Design review of the part built by this model. Coordinates are the model's own, in mm. A direction names the side the tool comes from. Coordinates: 2 decimals unless noted, no trailing zeros. Write each loop counter-clockwise with the first axis right and the second up, starting at its lowest first coordinate (ties: lowest second). Pieces come first, ordered by that corner, then holes. Notation, with made-up numbers: M 68.25,0 L 80.25,0 A29 cw 80.25,22 Z; hole C -36.75,30 d6. An arc over 180 degrees is marked long. One line per question, with ' | ' between items.
from build123d import *

# Parameters (mm, degrees)
SKETCH1_W               = 175
SKETCH1_H               = 80
BOSS_EXTRUDE1_DEPTH     = 7
SKETCH2_R               = 2
CUT_EXTRUDE1_DEPTH      = 10
SKETCH3_W               = 160
SKETCH3_H               = 52
CUT_EXTRUDE2_DEPTH      = 1
CUT_EXTRUDE3_DEPTH      = 10
SKETCH7_W               = 6
SKETCH7_H               = 15.226692755
SKETCH7_H_2             = 18
BOSS_EXTRUDE3_DEPTH     = 15
SKETCH8_R               = 2
CUT_EXTRUDE4_DEPTH      = 15
SKETCH9_W               = 20
SKETCH9_H               = 20
CUT_EXTRUDE5_DEPTH      = 15
SKETCH10_R              = 2
CUT_EXTRUDE7_DEPTH      = 51
CUT_EXTRUDE7_DEPTH_BACK = 31
SKETCH11_R              = 2
CUT_EXTRUDE8_DEPTH      = 10


with BuildPart() as part:
    # Sketch1 → Boss-Extrude1 (new body)
    with BuildSketch(Plane(origin=(0, 0, 0), x_dir=(1, 0, 0), z_dir=(0, 1, 0))):
        with Locations((-2.383449883, -6.993006993)):
            Rectangle(SKETCH1_W, SKETCH1_H)
    extrude(amount=BOSS_EXTRUDE1_DEPTH)

    # Sketch2 → Cut-Extrude1 (cut)
    with BuildSketch(Plane(origin=(0, 7, 0), x_dir=(1, 0, 0), z_dir=(0, 1, 0))):
        with Locations((-54.883449883, -32.893006993)):
            Circle(SKETCH2_R)
        with Locations((-2.383449883, -32.893006993)):
            Circle(SKETCH2_R)
        with Locations((50.116550117, -32.893006993)):
            Circle(SKETCH2_R)
    extrude(amount=-CUT_EXTRUDE1_DEPTH, mode=Mode.SUBTRACT)

    # Sketch3 → Cut-Extrude2 (cut)
    with BuildSketch(Plane(origin=(0, 7, 0), x_dir=(1, 0, 0), z_dir=(0, 1, 0))):
        with Locations((5.116550117, 7.006993007)):
            Rectangle(SKETCH3_W, SKETCH3_H)
    extrude(amount=-CUT_EXTRUDE2_DEPTH, mode=Mode.SUBTRACT)

    # Sketch6 → Cut-Extrude3 (cut)
    with BuildSketch(Plane(origin=(0, 6, 0), x_dir=(1, 0, 0), z_dir=(0, 1, 0))):
        Polygon((-70.883449883, 23.006993007), (-70.883449883, -18.993006993), (45.116550117, -18.993006993), (45.116550117, 23.006993007), (-9.883449883, 23.006993007), (-9.883449883, 28.006993007), (-70.883449883, 28.006993007), align=None)
    extrude(amount=-CUT_EXTRUDE3_DEPTH, mode=Mode.SUBTRACT)

    # Sketch7 → Boss-Extrude3 (add)
    with BuildSketch(Plane(origin=(0, 7, 0), x_dir=(1, 0, 0), z_dir=(0, 1, 0))):
        with Locations((-86.883449883, 25.39364663)):
            Rectangle(SKETCH7_W, SKETCH7_H)
        with Locations((-86.883449883, -32.993006993)):
            Rectangle(SKETCH7_W, SKETCH7_H_2)
    extrude(amount=BOSS_EXTRUDE3_DEPTH)

    # Sketch8 → Cut-Extrude4 (cut)
    with BuildSketch(Plane(origin=(-83.883449883, 0, 0), x_dir=(0, 0, -1), z_dir=(1, 0, 0))):
        with Locations((25.506993007, 14.5)):
            Circle(SKETCH8_R)
        with Locations((-32.993006993, 14.5)):
            Circle(SKETCH8_R)
    extrude(amount=-CUT_EXTRUDE4_DEPTH, mode=Mode.SUBTRACT)

    # Sketch9 → Cut-Extrude5 (cut)
    with BuildSketch(Plane.XZ):
        with Locations((75.116550117, 6.993006993)):
            Rectangle(SKETCH9_W, SKETCH9_H)
    extrude(amount=-CUT_EXTRUDE5_DEPTH, mode=Mode.SUBTRACT)

    # Sketch10 → Cut-Extrude7 (cut, two sides)
    with BuildSketch(Plane.XY.offset(-3.006993007)) as cut_extrude7_sk:
        with Locations((75.116550117, 3.5)):
            Circle(SKETCH10_R)
    extrude(amount=CUT_EXTRUDE7_DEPTH, mode=Mode.SUBTRACT)
    extrude(cut_extrude7_sk.sketch, amount=-CUT_EXTRUDE7_DEPTH_BACK, mode=Mode.SUBTRACT)

    # Sketch11 → Cut-Extrude8 (cut)
    with BuildSketch(Plane.XZ):
        with Locations((60.116550117, -23.006993007)):
            Circle(SKETCH11_R)
    extrude(amount=-CUT_EXTRUDE8_DEPTH, mode=Mode.SUBTRACT)


solid = part.part
1. Tool access review of faces 3 (the face through (-87, 14, 23.993)), 4 (the face through (-83.883, 12.7, -27)), 5 (the face through (-70.883, 3, -5)), 6 (the face through (28, 6, -24)): name each direction out of +Z, -Z, +X, -X, +Y, -Y from which nothing blocks a thin tool from reaching the whole face with its end or side.
Answer sheet:
face 3: +X, -X, +Y | face 4: +Z, -Z, +X, +Y | face 5: +Y, -Y | face 6: -Z, +X, +Y
2. Take a section at A-A (y = 9). Write out the cut boundary in (x, z).
Answer sheet:
outline: M -89.88,-33.01 L -83.88,-33.01 L -83.88,-17.78 L -89.88,-17.78 Z; M -89.88,23.99 L -83.88,23.99 L -83.88,41.99 L -89.88,41.99 Z
3. Take a section at B-B (x = -19). Write out the cut boundary in (y, z), then the cut area to 3 significant figures.
Answer sheet:
outline: M 0,-33.01 L 6,-33.01 L 6,-28.01 L 0,-28.01 Z; M 0,18.99 L 7,18.99 L 7,46.99 L 0,46.99 Z | area: 226 mm^2
4. To check wall thickness, follow line 1 along X through (y, z) = (2, 34.5); line 2 along X through (y, z) = (3, 9); line 3 along X through (y, z) = (12.75, -28). State the ranges of each line that lie inside material, in increasing order. Write a range as [from, to].
Answer sheet:
line 1: [-89.88, -56.07], [-53.69, -3.57], [-1.19, 48.93], [51.31, 73.79], [76.44, 85.12] | line 2: [-89.88, -70.88], [45.12, 65.12] | line 3: [-89.88, -83.88]
5. Draft analysis for pull direction Z (two halves, no side actions). For faces 1 (the face through (-14, 4, 18.993)), 2 (the face through (73.64, 4.85, 31.78)), state which applies: pulls with the +Z half, pulls with the -Z half, needs draft (parallel to the pull), parting line crosses it, or undercut.
Answer sheet:
face 1: undercut | face 2: needs draft
6. Insertion check: pin 1 Ø1.5 at (y, z) = (15, -19.5) entering from +X; pin 2 Ø1.8 at (x, y) = (-86, 11.5) entering from +Z; pin 3 Ø8 at (x, z) = (47.5, -17) entering from +Y. Each pin has a flat end and moves straight along its axis. Give the tip position at first contact, or say it passes through.
Answer sheet:
pin 1: x = -83.88 | pin 2: z = 41.99 | pin 3: y = 6
7. Take a section at C-C (z = 7.5). Write out the cut boundary in (x, y).
Answer sheet:
outline: M -89.88,0 L -70.88,0 L -70.88,6 L -74.88,6 L -74.88,7 L -89.88,7 Z; M 45.12,0 L 65.12,0 L 65.12,6 L 45.12,6 Z
